from build123d import *

# Parameters (mm, degrees)
F1_DEPTH = 6.35


with BuildPart() as f1:
    # F0 (on Right) → F1 (new body)
    with BuildSketch(Plane.YZ):
        Polygon((107.9963296652, 51.4815896749), (-114.268861711, 52.8442300856), (-114.268861711, 0), (107.9963296652, 0), align=None)
        with BuildLine():
            add(Edge.make_bspline(
                [(-30.0548927116, 16.0347425229), (-29.694553079, 15.2615137279), (-29.694553079, 14.2905986067)],
                knots=[0, 0, 0, 1, 1, 1], degree=2))
            add(Edge.make_bspline(
                [(-29.694553079, 14.2905986067), (-29.694553079, 11.8482966524), (-31.4236828438, 10.4795065202)],
                knots=[0, 0, 0, 1, 1, 1], degree=2))
            add(Edge.make_bspline(
                [(-31.4236828438, 10.4795065202), (-33.1528126086, 9.110716388), (-36.2957749597, 9.110716388)],
                knots=[0, 0, 0, 1, 1, 1], degree=2))
            add(Edge.make_bspline(
                [(-36.2957749597, 9.110716388), (-38.9382655988, 9.110716388), (-41.0652703746, 10.1917352858)],
                knots=[0, 0, 0, 1, 1, 1], degree=2))
            Line((-41.0652703746, 10.1917352858), (-41.0652703746, 12.6640655429))
            add(Edge.make_bspline(
                [(-41.0652703746, 12.6640655429), (-39.9692373254, 12.0084476002), (-38.7030438942, 11.6481079676)],
                knots=[0, 0, 0, 1, 1, 1], degree=2))
            add(Edge.make_bspline(
                [(-38.7030438942, 11.6481079676), (-37.436850463, 11.287768335), (-36.3558315651, 11.287768335)],
                knots=[0, 0, 0, 1, 1, 1], degree=2))
            add(Edge.make_bspline(
                [(-36.3558315651, 11.287768335), (-34.3889777372, 11.287768335), (-33.3880343132, 12.0685042057)],
                knots=[0, 0, 0, 1, 1, 1], degree=2))
            add(Edge.make_bspline(
                [(-33.3880343132, 12.0685042057), (-32.3870908893, 12.8492400763), (-32.3870908893, 14.0703910535)],
                knots=[0, 0, 0, 1, 1, 1], degree=2))
            add(Edge.make_bspline(
                [(-32.3870908893, 14.0703910535), (-32.3870908893, 14.9612307008), (-32.9326050554, 15.5718061894)],
                knots=[0, 0, 0, 1, 1, 1], degree=2))
            add(Edge.make_bspline(
                [(-32.9326050554, 15.5718061894), (-33.4781192214, 16.1823816779), (-35.2948315358, 17.2483864244)],
                knots=[0, 0, 0, 1, 1, 1], degree=2))
            add(Edge.make_bspline(
                [(-35.2948315358, 17.2483864244), (-37.3267466863, 18.3894619277), (-38.1725438795, 19.4829926183)],
                knots=[0, 0, 0, 1, 1, 1], degree=2))
            add(Edge.make_bspline(
                [(-38.1725438795, 19.4829926183), (-39.0183410727, 20.5765233089), (-39.0183410727, 22.0779384448)],
                knots=[0, 0, 0, 1, 1, 1], degree=2))
            add(Edge.make_bspline(
                [(-39.0183410727, 22.0779384448), (-39.0183410727, 24.2349715233), (-37.436850463, 25.5587192014)],
                knots=[0, 0, 0, 1, 1, 1], degree=2))
            add(Edge.make_bspline(
                [(-37.436850463, 25.5587192014), (-35.8553598532, 26.8824668795), (-33.2779305366, 26.8824668795)],
                knots=[0, 0, 0, 1, 1, 1], degree=2))
            add(Edge.make_bspline(
                [(-33.2779305366, 26.8824668795), (-30.6004068777, 26.8824668795), (-28.1130624692, 25.7213725078)],
                knots=[0, 0, 0, 1, 1, 1], degree=2))
            Line((-28.1130624692, 25.7213725078), (-28.9588596625, 23.5793535806))
            Line((-28.9588596625, 23.5793535806), (-29.8346851584, 23.9697215159))
            add(Edge.make_bspline(
                [(-29.8346851584, 23.9697215159), (-31.4161757681, 24.6453583271), (-33.2779305366, 24.6453583271)],
                knots=[0, 0, 0, 1, 1, 1], degree=2))
            add(Edge.make_bspline(
                [(-33.2779305366, 24.6453583271), (-34.7292985013, 24.6453583271), (-35.5600815431, 23.9647167988)],
                knots=[0, 0, 0, 1, 1, 1], degree=2))
            add(Edge.make_bspline(
                [(-35.5600815431, 23.9647167988), (-36.390864585, 23.2840752706), (-36.390864585, 22.2030563727)],
                knots=[0, 0, 0, 1, 1, 1], degree=2))
            add(Edge.make_bspline(
                [(-36.390864585, 22.2030563727), (-36.390864585, 21.3272308768), (-35.8353409847, 20.7016412369)],
                knots=[0, 0, 0, 1, 1, 1], degree=2))
            add(Edge.make_bspline(
                [(-35.8353409847, 20.7016412369), (-35.2798173844, 20.0760515969), (-33.543180544, 19.0901223244)],
                knots=[0, 0, 0, 1, 1, 1], degree=2))
            add(Edge.make_bspline(
                [(-33.543180544, 19.0901223244), (-31.8666003089, 18.154240223), (-31.1409163266, 17.4811057705)],
                knots=[0, 0, 0, 1, 1, 1], degree=2))
            add(Edge.make_bspline(
                [(-31.1409163266, 17.4811057705), (-30.4152323442, 16.8079713179), (-30.0548927116, 16.0347425229)],
                knots=[0, 0, 0, 1, 1, 1], degree=2))
        make_face(mode=Mode.SUBTRACT)
        with BuildLine():
            add(Edge.make_bspline(
                [(-21.7645788031, 25.3009762697), (-19.8102367679, 26.8824668795), (-17.4780385902, 26.8824668795)],
                knots=[0, 0, 0, 1, 1, 1], degree=2))
            add(Edge.make_bspline(
                [(-17.4780385902, 26.8824668795), (-16.0416847769, 26.8824668795), (-14.915623425, 26.106735726)],
                knots=[0, 0, 0, 1, 1, 1], degree=2))
            add(Edge.make_bspline(
                [(-14.915623425, 26.106735726), (-13.7895620731, 25.3310045725), (-13.1639724332, 23.8796366078)],
                knots=[0, 0, 0, 1, 1, 1], degree=2))
            Line((-13.1639724332, 23.8796366078), (-12.988807334, 23.8796366078))
            Line((-12.988807334, 23.8796366078), (-11.942821456, 26.567169701))
            Line((-11.942821456, 26.567169701), (-9.9559487595, 26.567169701))
            Line((-9.9559487595, 26.567169701), (-13.5993828226, 9.4260135666))
            Line((-13.5993828226, 9.4260135666), (-15.6813451443, 9.4260135666))
            Line((-15.6813451443, 9.4260135666), (-15.2709583405, 12.6940938456))
            Line((-15.2709583405, 12.6940938456), (-15.3960762685, 12.6940938456))
            add(Edge.make_bspline(
                [(-15.3960762685, 12.6940938456), (-18.1987178554, 9.110716388), (-21.2966377524, 9.110716388)],
                knots=[0, 0, 0, 1, 1, 1], degree=2))
            add(Edge.make_bspline(
                [(-21.2966377524, 9.110716388), (-23.4686849823, 9.110716388), (-24.7048501108, 10.6596763365)],
                knots=[0, 0, 0, 1, 1, 1], degree=2))
            add(Edge.make_bspline(
                [(-24.7048501108, 10.6596763365), (-25.9410152394, 12.208636285), (-25.9410152394, 14.9011740953)],
                knots=[0, 0, 0, 1, 1, 1], degree=2))
            add(Edge.make_bspline(
                [(-25.9410152394, 14.9011740953), (-25.9410152394, 18.154240223), (-24.8299680388, 20.9368629415)],
                knots=[0, 0, 0, 1, 1, 1], degree=2))
            add(Edge.make_bspline(
                [(-24.8299680388, 20.9368629415), (-23.7189208383, 23.71948566), (-21.7645788031, 25.3009762697)],
                knots=[0, 0, 0, 1, 1, 1], degree=2))
        make_face(mode=Mode.SUBTRACT)
        Polygon((-45.9598837175, 9.4260135666), (-48.5873602053, 9.4260135666), (-43.7227751651, 32.2925660857), (-41.0952986773, 32.2925660857), align=None, mode=Mode.SUBTRACT)
        with BuildLine():
            add(Edge.make_bspline(
                [(19.2916180871, 9.3859758296), (18.1655567352, 9.110716388), (16.8092783958, 9.110716388)],
                knots=[0, 0, 0, 1, 1, 1], degree=2))
            add(Edge.make_bspline(
                [(16.8092783958, 9.110716388), (13.931566052, 9.110716388), (12.2875164783, 10.8173249258)],
                knots=[0, 0, 0, 1, 1, 1], degree=2))
            add(Edge.make_bspline(
                [(12.2875164783, 10.8173249258), (10.6434669045, 12.5239334636), (10.6434669045, 15.5417778866)],
                knots=[0, 0, 0, 1, 1, 1], degree=2))
            add(Edge.make_bspline(
                [(10.6434669045, 15.5417778866), (10.6434669045, 18.4795468358), (11.8095659933, 21.1795917218)],
                knots=[0, 0, 0, 1, 1, 1], degree=2))
            add(Edge.make_bspline(
                [(11.8095659933, 21.1795917218), (12.9756650822, 23.8796366078), (14.8999788147, 25.3810517437)],
                knots=[0, 0, 0, 1, 1, 1], degree=2))
            add(Edge.make_bspline(
                [(14.8999788147, 25.3810517437), (16.8242925471, 26.8824668795), (19.1364718564, 26.8824668795)],
                knots=[0, 0, 0, 1, 1, 1], degree=2))
            add(Edge.make_bspline(
                [(19.1364718564, 26.8824668795), (21.5287266395, 26.8824668795), (22.7348634653, 25.8414857187)],
                knots=[0, 0, 0, 1, 1, 1], degree=2))
            add(Edge.make_bspline(
                [(22.7348634653, 25.8414857187), (23.9410002911, 24.8005045578), (23.9410002911, 22.9387497893)],
                knots=[0, 0, 0, 1, 1, 1], degree=2))
            add(Edge.make_bspline(
                [(23.9410002911, 22.9387497893), (23.9410002911, 20.1260987681), (21.3435521061, 18.5220869313)],
                knots=[0, 0, 0, 1, 1, 1], degree=2))
            add(Edge.make_bspline(
                [(21.3435521061, 18.5220869313), (18.746103921, 16.9180750945), (13.9115471835, 16.9180750945)],
                knots=[0, 0, 0, 1, 1, 1], degree=2))
            Line((13.9115471835, 16.9180750945), (13.3960613202, 16.9180750945))
            Line((13.3960613202, 16.9180750945), (13.3360047148, 15.6668958146))
            add(Edge.make_bspline(
                [(13.3360047148, 15.6668958146), (13.3360047148, 13.6199665127), (14.2969104018, 12.4688815752)],
                knots=[0, 0, 0, 1, 1, 1], degree=2))
            add(Edge.make_bspline(
                [(14.2969104018, 12.4688815752), (15.2578160887, 11.3177966377), (17.2747170879, 11.3177966377)],
                knots=[0, 0, 0, 1, 1, 1], degree=2))
            add(Edge.make_bspline(
                [(17.2747170879, 11.3177966377), (18.2606463604, 11.3177966377), (19.3016275213, 11.600563155)],
                knots=[0, 0, 0, 1, 1, 1], degree=2))
            add(Edge.make_bspline(
                [(19.3016275213, 11.600563155), (20.3426086822, 11.8833296722), (21.8890662721, 12.6340372402)],
                knots=[0, 0, 0, 1, 1, 1], degree=2))
            Line((21.8890662721, 12.6340372402), (21.8890662721, 10.3468815165))
            add(Edge.make_bspline(
                [(21.8890662721, 10.3468815165), (20.417679439, 9.6612352712), (19.2916180871, 9.3859758296)],
                knots=[0, 0, 0, 1, 1, 1], degree=2))
        make_face(mode=Mode.SUBTRACT)
        with BuildLine():
            add(Edge.make_bspline(
                [(3.4717072722, 10.6671834122), (1.5549006154, 9.110716388), (-0.8523683191, 9.110716388)],
                knots=[0, 0, 0, 1, 1, 1], degree=2))
            add(Edge.make_bspline(
                [(-0.8523683191, 9.110716388), (-2.3687976063, 9.110716388), (-3.5173801853, 9.9089687686)],
                knots=[0, 0, 0, 1, 1, 1], degree=2))
            add(Edge.make_bspline(
                [(-3.5173801853, 9.9089687686), (-4.6659627642, 10.7072211492), (-5.2465099501, 12.083518357)],
                knots=[0, 0, 0, 1, 1, 1], degree=2))
            Line((-5.2465099501, 12.083518357), (-5.4016561808, 12.083518357))
            Line((-5.4016561808, 12.083518357), (-6.4976892299, 9.4260135666))
            Line((-6.4976892299, 9.4260135666), (-8.4545336237, 9.4260135666))
            Line((-8.4545336237, 9.4260135666), (-3.2896655563, 33.7639529189))
            Line((-3.2896655563, 33.7639529189), (-0.6621890686, 33.7639529189))
            add(Edge.make_bspline(
                [(-0.6621890686, 33.7639529189), (-1.4629438077, 29.9753820594), (-1.89334948, 27.9659881359)],
                knots=[0, 0, 0, 1, 1, 1], degree=2))
            add(Edge.make_bspline(
                [(-1.89334948, 27.9659881359), (-2.3237551522, 25.9565942124), (-3.0744627202, 23.2690611192)],
                knots=[0, 0, 0, 1, 1, 1], degree=2))
            Line((-3.0744627202, 23.2690611192), (-2.9293259237, 23.2690611192))
            add(Edge.make_bspline(
                [(-2.9293259237, 23.2690611192), (-1.477957959, 25.1107970192), (-0.0616230142, 25.9791154394)],
                knots=[0, 0, 0, 1, 1, 1], degree=2))
            add(Edge.make_bspline(
                [(-0.0616230142, 25.9791154394), (1.3547119306, 26.8474338597), (2.8561270665, 26.8474338597)],
                knots=[0, 0, 0, 1, 1, 1], degree=2))
            add(Edge.make_bspline(
                [(2.8561270665, 26.8474338597), (5.0582025991, 26.8474338597), (6.2943677276, 25.3009762697)],
                knots=[0, 0, 0, 1, 1, 1], degree=2))
            add(Edge.make_bspline(
                [(6.2943677276, 25.3009762697), (7.5305328561, 23.7545186798), (7.5305328561, 21.0469667181)],
                knots=[0, 0, 0, 1, 1, 1], degree=2))
            add(Edge.make_bspline(
                [(7.5305328561, 21.0469667181), (7.5305328561, 17.7788864391), (6.4595233926, 15.0012684377)],
                knots=[0, 0, 0, 1, 1, 1], degree=2))
            add(Edge.make_bspline(
                [(6.4595233926, 15.0012684377), (5.388513929, 12.2236504364), (3.4717072722, 10.6671834122)],
                knots=[0, 0, 0, 1, 1, 1], degree=2))
        make_face(mode=Mode.SUBTRACT)
        Polygon((33.6201232003, 33.7639529189), (28.4252268302, 9.4260135666), (25.7977503425, 9.4260135666), (30.9926467125, 33.7639529189), align=None, mode=Mode.SUBTRACT)
    extrude(amount=F1_DEPTH)


solid = f1.part
Check sheet for the modelled part. Datum: model origin and axes. Units: mm. A direction names the side the tool comes from. Round coordinates to 2 decimals unless told otherwise and drop trailing zeros. Loops run counter-clockwise (first coordinate to the right, second up) from the corner with the lowest first, then second, coordinate; pieces in that order, holes last. Notation, with made-up numbers: M -32,-16 L -4,-16 A15 cw -4,8 Z; hole C 55.25,38 d3. An arc over 180 degrees is marked long. One line per item, written item: value.
(1) Release check for a two-part mould opening along Y. For faces 1 (the face through (3, -114.269, 27)), 2 (the face through (6.35, -5, 33)), 3 (the face through (3.13, -11.75, 18.12)) record: +Y half, -Y half, draft (parallel to the pull), parting line (faces both ways), or undercut.
Computed values:
face 1: -Y half
face 2: draft
face 3: undercut
(2) Access from +Z, -Z, +X, -X, +Y, -Y to the whole of each face (thin tool, end or side, straight path). Record for faces 4 (the face through (3, -6, 21)), 5 (the face through (3, 107.996, 25)).
Computed values:
face 4: +X, -X
face 5: +Z, -Z, +X, -X, +Y
(3) Depth check by flat-ended pin: pin 1 Ø1 at (x, y) = (1, 12) entering from +Z; pin 2 Ø2.5 at (x, y) = (3, -15) entering from +Z; pin 3 Ø2 at (x, y) = (4, -48) entering from +Z. Enter the tip coordinate at first touch or a pass-through.
Computed values:
pin 1: stops at z = 52.07
pin 2: stops at z = 52.24
pin 3: stops at z = 52.44
(4) Thickness scan on line 1 (Y direction, x = 2.25, z = 32.5); line 2 (Y direction, x = 1.5, z = 33); line 3 (Z direction, x = 1, y = 40.5). Record the ranges inside material, lowest first.
Computed values:
line 1: y = -114.27 to -3.56, -0.93 to 30.72, 33.35 to 108
line 2: y = -114.27 to -3.45, -0.82 to 30.83, 33.46 to 108
line 3: z = 0 to 51.9
(5) Sectioned sample at A-A, the plane x = 1.5. Count the separate pieces of the cut face and the enclosed holes in it, then the cut area to 3 significant figures.
Computed values:
separate pieces: 1
enclosed holes: 6
area: 10,800 mm^2
(6) Sectioned sample at B-B, the plane y = 83. Record the cut outline in (x, z).
Computed values:
outline: M 0,0 L 6.35,0 L 6.35,51.63 L 0,51.63 Z
